Autodesk Inventor part; units mm, degrees
ref_plane "YZ Plane" through (0, 0, 0) normal (1, 0, 0) x (0, 1, 0)
ref_plane "XZ Plane" through (0, 0, 0) normal (0, 1, 0) x (-1, 0, 0)
ref_plane "XY Plane" through (0, 0, 0) normal (0, 0, 1) x (1, 0, 0)
sketch "Skizze1" plane through (0, 0, 0) normal (0, 0, 1) x (1, 0, 0)
  line L0 (13, 0) -> (0, 0)
  line L1 (0, 0) -> (0, 21)
  line L2 (0, 21) -> (4, 21)
  line L3 (4, 21) -> (4, 30)
  line L4 (4, 30) -> (0, 30)
  line L5 (0, 30) -> (0, 51)
  line L6 (0, 51) -> (13, 51)
  line L7 (13, 51) -> (21, 43)
  line L8 (21, 43) -> (21, 30)
  line L9 (21, 30) -> (27, 30)
  line L10 (27, 30) -> (27, 43)
  line L11 (27, 43) -> (35, 51)
  line L12 (35, 51) -> (48, 51)
  line L13 (48, 51) -> (48, 30)
  line L14 (48, 30) -> (44, 30)
  line L15 (44, 30) -> (44, 21)
  line L16 (44, 21) -> (48, 21)
  line L17 (48, 21) -> (48, 0)
  line L18 (48, 0) -> (35, 0)
  line L19 (35, 0) -> (27, 8)
  line L20 (27, 8) -> (27, 13)
  line L21 (27, 13) -> (21, 13)
  line L22 (21, 13) -> (21, 8)
  line L23 (21, 8) -> (13, 0)
  point P0 (48, 40.5)
  point P1 (41.5, 51)
  dimension "d0" = 21
  dimension "d1" = 9
  dimension "d2" = 21
  dimension "d3" = 21
  dimension "d4" = 21
  dimension "d5" = 4
  dimension "d6" = 4
  dimension "d7" = 13
  dimension "d8" = 22
  dimension "d9" = 13
  dimension "d10" = 21
  dimension "d11" = 135
  dimension "d12" = 135
  dimension "d13" = 45
  dimension "d14" = 45
extrude "Extrusion1" add sketch "Skizze1" against normal blind 10
equation "\"d2\" = d0"
equation "\"d4\" = d3"
equation "\"d14\" = d13"
properties part number "Vblock"
The model under review builds one solid part; all positions refer to its coordinate system, in mm. A direction names the side the tool comes from. Round coordinates to 2 decimals unless told otherwise and drop trailing zeros. Write each loop counter-clockwise with the first axis right and the second up, starting at its lowest first coordinate (ties: lowest second). Pieces come first, ordered by that corner, then holes. Notation, with made-up numbers: M 39.5,77 L 55.5,77 A19 cw 55.5,97 Z; hole C 79.25,-17.75 d7. An arc over 180 degrees is marked long. Use a Markdown table: item, result. Add a question column.
Q1. We need section A-A, the plane y = 39. State the section outline as (x, z) points, plus the area to 3 significant figures.
Q2. Insertion check: pin 1 (3 mm diameter, centred on x = 25, z = -4, fed in from +Y); pin 2 (5 mm diameter, centred on x = 25, z = -6.5, fed in from -Y); pin 3 (2.5 mm diameter, centred on y = 26.5, z = -7.5, fed in from -X). Each pin has a flat end and moves straight along its axis. Give the tip position at first contact, or say it passes through.
Q3. The part is to be moulded in two halves that separate along X. For faces 5 (the face through (7, 0, -5)), 6 (the face through (27, 10, -5)), 7 (the face through (48, 11, -5)), say which applies: pulls with the +X half, pulls with the -X half, needs draft (parallel to the pull), parting line crosses it, or undercut.
Q4. Machinability: for faces 1 (the face through (17, 4, -5)), 2 (the face through (44, 26, -5)), 3 (the face through (2, 21, -5)), 4 (the face through (21, 37, -5)), which of the approach directions +Z, -Z, +X, -X, +Y, -Y give a long, thin tool a straight path to every point of the face, cutting with its end or side? Answer none if there is none.
Q5. We need section B-B, the plane z = -6. State the section outline as (x, y) points, plus the area to 3 significant figures.
Q6. We need section D-D, the plane x = 23. State the section outline as (y, z) points, plus the area to 3 significant figures.
Q7. To check wall thickness, follow line 1 (Y direction, x = 44.5, z = -8); line 2 (X direction, y = 21.5, z = -2.25); line 3 (X direction, y = 40.5, z = -0.75). State the ranges of each line that lie inside material, in increasing order.
Q8. We need section C-C, the plane y = 3. State the section outline as (x, z) points, plus the area to 3 significant figures.
Findings below:
| question | item | result |
|---|---|---|
| 1 | outline | M 0,-10 L 21,-10 L 21,0 L 0,0 Z; M 27,-10 L 48,-10 L 48,0 L 27,0 Z |
| 1 | area | 420 mm² |
| 2 | pin 1 | stops at y = 30 |
| 2 | pin 2 | stops at y = 7.5 |
| 2 | pin 3 | stops at x = 4 |
| 3 | face 5 | needs draft |
| 3 | face 6 | undercut |
| 3 | face 7 | pulls with the +X half |
| 4 | face 1 | +Z, -Z, -Y |
| 4 | face 2 | +Z, -Z, +X |
| 4 | face 3 | +Z, -Z, -X |
| 4 | face 4 | +Z, -Z, +Y |
| 5 | outline | M 0,0 L 13,0 L 21,8 L 21,13 L 27,13 L 27,8 L 35,0 L 48,0 L 48,21 L 44,21 L 44,30 L 48,30 L 48,51 L 35,51 L 27,43 L 27,30 L 21,30 L 21,43 L 13,51 L 0,51 L 0,30 L 4,30 L 4,21 L 0,21 Z |
| 5 | area | 2,040 mm² |
| 6 | outline | M 13,-10 L 30,-10 L 30,0 L 13,0 Z |
| 6 | area | 170 mm² |
| 7 | line 1 | y = 0 to 21, 30 to 51 |
| 7 | line 2 | x = 4 to 44 |
| 7 | line 3 | x = 0 to 21, 27 to 48 |
| 8 | outline | M 0,-10 L 16,-10 L 16,0 L 0,0 Z; M 32,-10 L 48,-10 L 48,0 L 32,0 Z |
| 8 | area | 320 mm² |
